Answer from the drawing. Dimensions are ordinates in mm from the lowest x, y and z of the part. A direction names the side the tool comes from. Coordinates: 2 decimals unless noted, no trailing zeros. Write each loop counter-clockwise with the first axis right and the second up, starting at its lowest first coordinate (ties: lowest second). Pieces come first, ordered by that corner, then holes. Notation, with made-up numbers: (46.25, 39) - (100.25, 39) arc R16 cw to (100.25, 67) - close; hole circle Ø9 at (48.5, 37.25). An arc over 180 degrees is marked (long way). Return JSON: item names as keys, results as strings.
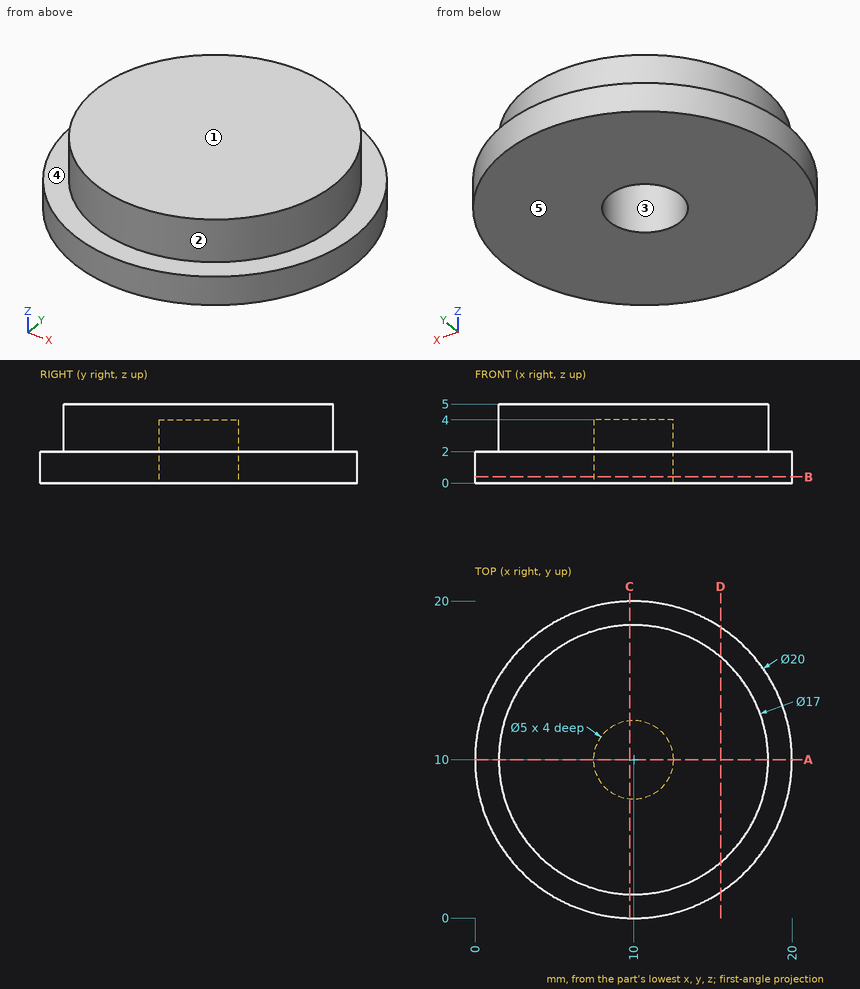
(1) A cutting plane is placed at D-D (x = 15.5). Determine the outline of the cut face in (y, z), and give its area (3 significant figures).
Answer:
{"outline": "(1.65, 0) - (18.35, 0) - (18.35, 2) - (16.48, 2) - (16.48, 5) - (3.52, 5) - (3.52, 2) - (1.65, 2) - close", "area": "72.3 mm²"}
(2) Determine the mould class of the marked faces 1, 2 and 3 for opening direction X: +X half, -X half, draft (parallel to the pull), parting line (faces both ways), or undercut.
Answer:
{"face 1": "draft", "face 2": "parting line", "face 3": "undercut"}
(3) A cutting plane is placed at A-A (y = 10). Determine the outline of the cut face in (x, z).
Answer:
{"outline": "(0, 0) - (7.5, 0) - (7.5, 4) - (12.5, 4) - (12.5, 0) - (20, 0) - (20, 2) - (18.5, 2) - (18.5, 5) - (1.5, 5) - (1.5, 2) - (0, 2) - close"}
(4) Which of the six approach directions +Z, -Z, +X, -X, +Y, -Y give full straight-line access (tool end or side, diameter ignored) to the marked faces 4 and 5?
Answer:
{"face 4": "+Z", "face 5": "-Z, +X, -X, +Y, -Y"}
(5) A cutting plane is placed at B-B (z = 0.4). Determine the outline of the cut face in (x, y), and give its area (3 significant figures).
Answer:
{"outline": "circle Ø20 at (10, 10); hole circle Ø5 at (10, 10)", "area": "295 mm²"}
(6) A cutting plane is placed at C-C (x = 9.75). Determine the outline of the cut face in (y, z), and give its area (3 significant figures).
Answer:
{"outline": "(0, 0) - (7.51, 0) - (7.51, 4) - (12.49, 4) - (12.49, 0) - (20, 0) - (20, 2) - (18.5, 2) - (18.5, 5) - (1.5, 5) - (1.5, 2) - (0, 2) - close", "area": "71.1 mm²"}
(7) Straight lines are drawn through the part: line 1 (Y direction, x = 10, z = 3.05); line 2 (Z direction, x = 4.5, y = 1.75); line 3 (Y direction, x = 7.75, z = 2.95). For each, find the intervals that lie inside material, in ascending order. Write a range as from..to.
Answer:
{"line 1": "1.5..7.5, 12.5..18.5", "line 2": "0..2", "line 3": "1.8..8.91, 11.09..18.2"}
(8) Flat-ended cylindrical pins translate along their axes: P1, Ø2, axis at x = 12, z = 1.5, coming from the -Y side; P2, Ø1.5, axis at x = 5, z = 3, coming from the +Y side; P3, Ø1.5, axis at x = 10.5, y = 10, coming from the -Z side. Find the tip coordinate at first contact, or state that the pin passes through.
Answer:
{"P1": "y = 0.05", "P2": "y = 17.36", "P3": "z = 4"}
